Geometry check sheet. Reference: the model listing, model coordinates, mm. A direction names the side the tool comes from. Coordinates: 2 decimals unless noted, no trailing zeros. Loops run counter-clockwise (first coordinate to the right, second up) from the corner with the lowest first, then second, coordinate; pieces in that order, holes last. Notation, with made-up numbers: (4, 78.25) - (17, 78.25) arc R5 cw to (17, 85.25) - close; hole circle Ø4 at (61, 88.25). An arc over 180 degrees is marked (long way). Write item = value, one per line. Start each with the question number.
Autodesk Inventor part; units mm, degrees
ref_plane "YZ Plane" through (0, 0, 0) normal (1, 0, 0) x (0, 1, 0)
ref_plane "XZ Plane" through (0, 0, 0) normal (0, 1, 0) x (-1, 0, 0)
ref_plane "XY Plane" through (0, 0, 0) normal (0, 0, 1) x (1, 0, 0)
sketch "Sketch1" plane through (0, 0, 0) normal (0, 0, 1) x (1, 0, 0)
  line L0 (-60, 75) -> (60, 75)
  line L1 (60, 75) -> (60, -75)
  line L2 (60, -75) -> (-60, -75)
  line L3 (-60, -75) -> (-60, 75)
  point P0 (0, 0)
  point P1 (60, 0)
  point P2 (0, 75)
  dimension "d0" = 120
  dimension "d1" = 150
extrude "Extrusion1" add sketch "Sketch1" along normal blind 6
sketch "Sketch2" plane through (0, 0, 6) normal (0, 0, 1) x (1, 0, 0)
  line L0 (-37.3514, 35.3082) -> (6.6486, 35.3082)
  line L1 (6.6486, 35.3082) -> (6.6486, -8.6918)
  line L2 (6.6486, -8.6918) -> (-37.3514, -8.6918)
  line L3 (-37.3514, -8.6918) -> (-37.3514, 35.3082)
  point P0 (0, 0)
  dimension "d4" = 44
  dimension "d5" = 44
extrude "Hole" cut sketch "Sketch2" against normal through all
sketch "Sketch3" plane through (0, 0, 6) normal (0, 0, 1) x (1, 0, 0)
  line L0 (6.6486, 35.3082) -> (6.6486, -8.6918)
  line L1 (6.6486, -8.6918) -> (-37.3514, -8.6918)
  line L2 (-37.3514, -8.6918) -> (-37.3514, 35.3082)
  line L3 (-37.3514, 35.3082) -> (6.6486, 35.3082)
  line L4 (-60, -75) -> (60, -75)
  line L5 (60, -75) -> (60, 75)
  line L6 (60, 75) -> (-60, 75)
  line L7 (-60, 75) -> (-60, -75)
  line L8 (-60, 9.6891) -> (-42.5, 75)
  line L9 (42.5, 75) -> (60, 9.6891)
  line L10 (-42.5, 75) -> (42.5, 75)
  line L11 (60, 75) -> (-60, 75) construction
  point P0 (0, 0)
  point P1 (0, 75)
  dimension "d9" = 15
  dimension "d10" = 85
extrude "Extrusion3" cut sketch "Sketch3" against normal through all contours L7 L6 L8 | L9 L6 L5
fillet "Fillet1" radius 10 4 edges at (60, -75, 3) (-60, -75, 3) (-42.5, 75, 3) (42.5, 75, 3)
fillet "Fillet2" radius 100 2 edges at (60, 9.6891, 3) (-60, 9.6891, 3)
chamfer "Chamfer1" distance 0.5 angle 45 24 edges at (0, 75, 6) (-40.9143, 72.9335, 6) (-50.5393, 44.997, 6) (-59.1445, 9.5765, 6) (-60, -34.2381, 6) (-57.0711, -72.0711, 6) (0, -75, 6) (57.0711, -72.0711, 6) (60, -34.2381, 6) (59.1445, 9.5765, 6) (50.5393, 44.997, 6) (40.9143, 72.9335, 6) (0, 75, 0) (-40.9143, 72.9335, 0) (-50.5393, 44.997, 0) (-59.1445, 9.5765, 0) (-60, -34.2381, 0) (-57.0711, -72.0711, 0) (0, -75, 0) (57.0711, -72.0711, 0) (60, -34.2381, 0) (59.1445, 9.5765, 0) (50.5393, 44.997, 0) (40.9143, 72.9335, 0)
equation "\"d0\" = width"
equation "\"d1\" = hight"
equation "\"hight\" = 150"
equation "\"width\" = 120"
properties part number "tc-front-panel" material "ABS Plastic"
(1) Sectioned sample at D-D on y = 46. Enter the section's corners in (x, z).
(2) Sectioned sample at B-B on z = 3.5. Enter the section's corners in (x, y), plus the area to 3 significant figures.
(3) Draft check along Y on faces 3 (the face through (-50.216, 45.249, 0.254)), 4 (the face through (-16, 35.308, 3)), 5 (the face through (-15, -8.692, 3)), 6 (the face through (-1, -16, 6)). Enter one of: pulls with the +Y half, pulls with the -Y half, needs draft (parallel to the pull), parting line crosses it, or undercut.
(4) Depth check by flat-ended pin: pin 1 (1.8 mm diameter, centred on y = 5, z = 1.5, fed in from +X); pin 2 (1 mm diameter, centred on y = 43.5, z = 2, fed in from -X). Enter the tip coordinate at first touch or a pass-through.
(5) Sectioned sample at C-C on y = 26.5. Enter the section's corners in (x, z).
(6) Tool access check on faces 1 (the face through (40.84, 72.99, 2.96)), 2 (the face through (-37.351, 13, 3)). Record the directions out of +Z, -Z, +X, -X, +Y, -Y that give a thin tool (end or side, any length) a straight path to the whole face; none if there is none.
(7) Sectioned sample at A-A on x = -8. Enter the section's corners in (y, z), plus the area to 4 significant figures.
(8) Scan lines: line 1 (Y direction, x = -30, z = 5.5); line 2 (X direction, y = 0, z = 1); line 3 (X direction, y = 14, z = 4.25). Record each from-to range of solid material in increasing order.
Working result:
q1.outline = (-50.27, 0.5) - (-49.75, 0) - (49.75, 0) - (50.27, 0.5) - (50.27, 5.5) - (49.75, 6) - (-49.75, 6) - (-50.27, 5.5) - close
q2.outline = (-60, -65) arc R10 ccw to (-50, -75) - (50, -75) arc R10 ccw to (60, -65) - (60, -3.48) arc R100 ccw to (56.59, 22.41) - (44.49, 67.59) arc R10 ccw to (34.83, 75) - (-34.83, 75) arc R10 ccw to (-44.49, 67.59) - (-56.59, 22.41) arc R100 ccw to (-60, -3.48) - close; hole (-37.35, -8.69) - (6.65, -8.69) - (6.65, 35.31) - (-37.35, 35.31) - close
q2.area = 14,800 mm2
q3.face_3 = pulls with the +Y half
q3.face_4 = undercut
q3.face_5 = undercut
q3.face_6 = needs draft
q4.pin_1 = 59.71
q4.pin_2 = -51.07
q5.outline = (-55.5, 0.5) - (-54.98, 0) - (-37.35, 0) - (-37.35, 6) - (-54.98, 6) - (-55.5, 5.5) - close; (6.65, 0) - (54.98, 0) - (55.5, 0.5) - (55.5, 5.5) - (54.98, 6) - (6.65, 6) - close
q6.face_1 = +Z, -Z, +X, +Y
q6.face_2 = +Z, -Z
q7.outline = (-75, 0.5) - (-74.5, 0) - (-8.69, 0) - (-8.69, 6) - (-74.5, 6) - (-75, 5.5) - close; (35.31, 0) - (74.5, 0) - (75, 0.5) - (75, 5.5) - (74.5, 6) - (35.31, 6) - close
q7.area = 635.5 mm2
q8.line_1 = -75 to -8.69, 35.31 to 75
q8.line_2 = -59.94 to -37.35, 6.65 to 59.94
q8.line_3 = -58.46 to -37.35, 6.65 to 58.46
